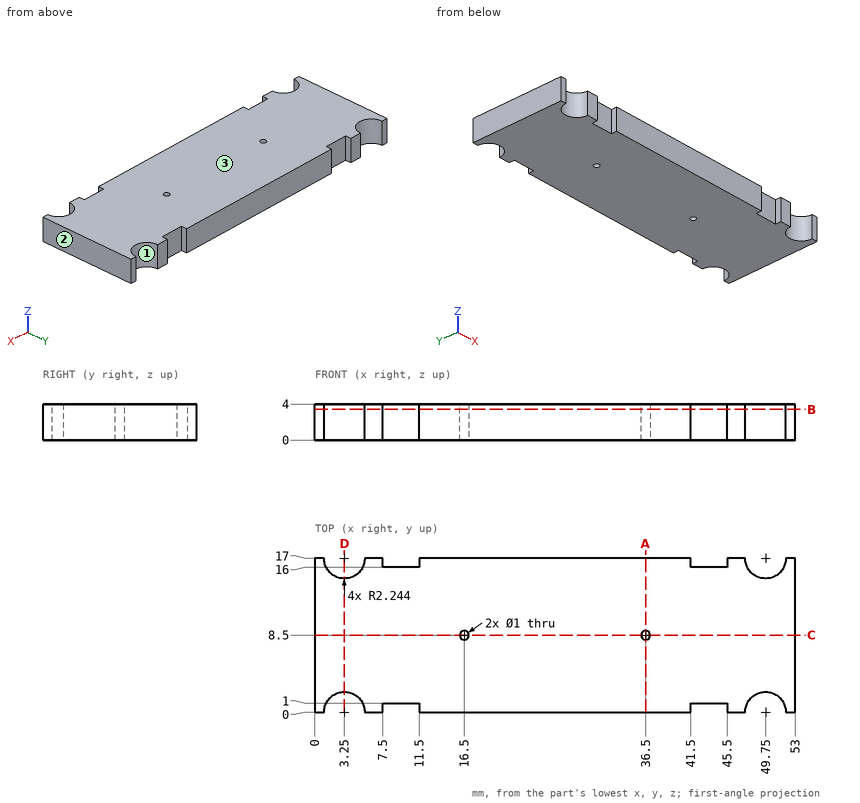
Geometry check sheet. Reference: drawing and pictorial views, mm from the part's lowest x, y, z. Round coordinates to 2 decimals unless told otherwise and drop trailing zeros. Order: outer loops, then holes, each group sorted by start corner. A loop starts at its lowest first (then second) coordinate and runs counter-clockwise, first axis right, second up. Notation, with made-up numbers: (-33, -33.75) - (-21, -33.75) arc R14 cw to (-21, -21.75) - close; hole circle Ø11 at (49.5, 2). An arc over 180 degrees is marked (long way). Write item = value, one per line.
Q1. Section check A-A (x = 36.5). Record the boundary of the cut face in (y, z).
Computed:
outline = (0, 0) - (8, 0) - (8, 4) - (0, 4) - close; (9, 0) - (17, 0) - (17, 4) - (9, 4) - close
Q2. Section check B-B (z = 3.4). State how many separate pieces and enclosed holes the cut face has, and give its area (3 significant figures).
Computed:
separate_pieces = 1
enclosed_holes = 2
area = 852 mm^2
Q3. Section check C-C (y = 8.5). Record the boundary of the cut face in (x, z), and give its area (3 significant figures).
Computed:
outline = (0, 0) - (16, 0) - (16, 4) - (0, 4) - close; (17, 0) - (36, 0) - (36, 4) - (17, 4) - close; (37, 0) - (53, 0) - (53, 4) - (37, 4) - close
area = 204 mm^2
Q4. Draft check along X on the marked faces 1, 2 and 3. Enter one of: pulls with the +X half, pulls with the -X half, needs draft (parallel to the pull), parting line crosses it, or undercut.
Computed:
face_1 = undercut
face_2 = pulls with the +X half
face_3 = needs draft
Q5. Go/stop test with a flat-tipped pin: pin 1 (1.2 mm diameter, centred on x = 44.5, z = 1, fed in from +Y). Record where the tip stops, or that it passes through.
Computed:
pin_1 = 16
Q6. Section check D-D (x = 3.25). Record the boundary of the cut face in (y, z).
Computed:
outline = (2.24, 0) - (14.76, 0) - (14.76, 4) - (2.24, 4) - close
Q7. Thickness scan on line 1 along Y through (x, z) = (16.5, 1.9); line 2 along X through (y, z) = (15, 2.6) (1 decimal); line 3 along X through (y, z) = (8.25, 2.75). Record the ranges inside material, lowest first.
Computed:
line_1 = 0 to 8, 9 to 17
line_2 = 0 to 2.2, 4.3 to 48.7, 50.8 to 53
line_3 = 0 to 16.07, 16.93 to 36.07, 36.93 to 53
